Can you work these out from the model? Positions are in its coordinate system, mm. A direction names the side the tool comes from. Coordinates: 2 decimals unless noted, no trailing zeros. Order: outer loops, then holes, each group sorted by start corner. A loop starts at its lowest first (then second) coordinate and runs counter-clockwise, first axis right, second up. Notation, with made-up numbers: (-37.5, 54) -> (10.5, 54) arc R29 ccw to (10.5, 74) -> close; hole circle Ø11 at (63, 38.5). An arc over 180 degrees is marked (long way). Answer in a Markdown table with one row per item. Add a question column.
1. Imagine slicing it at C-C on x = -34. Write out the boundary of the cut face in (y, z), plus the area to 3 significant figures.
2. We'd pull the mould along Y, two halves only. Please class faces 1 (the face through (-22.185, -10.345, 0.21)), 2 (the face through (3.054, 2.707, 5.088)), 3 (the face through (-27, -18, 0)): pulls with the +Y half, pulls with the -Y half, needs draft (parallel to the pull), parting line crosses it, or undercut.
3. Imagine slicing it at B-B on y = 10. Write out the boundary of the cut face in (x, z), plus the area to 3 significant figures.
4. Will these pins go through, and if not, where does the flat tip stop? pin 1 (1.5 mm diameter, centred on x = -3, z = 3, fed in from +Y); pin 2 (5 mm diameter, centred on y = 14.71, z = -5, fed in from -X); pin 3 (3 mm diameter, centred on x = -12, y = -3.5, fed in from -Z); pin 4 (5 mm diameter, centred on y = -4.5, z = -2.5, fed in from -X).
5. If I drill on line 1 along X through (y, z) = (1, -10); line 2 along Z through (x, y) = (-25, -17.15); line 3 along Y through (x, z) = (-13.5, 12.5), over which ranges is the centre line in solid material (lowest first)? Write a range as [from, to].
6. Imagine slicing it at A-A on z = -10.25. Write out the boundary of the cut face in (x, y).
7. On a 3-axis mill with a long thin cutter (end or side, diameter ignored), from which of +Z, -Z, +X, -X, +Y, -Y can I reach the whole of each face in a straight line? I mean faces 4 (the face through (-9, -8, -15)), 5 (the face through (-4.53, -9.83, 6.77)), 6 (the face through (0, -18, 2)). Say none if no direction works.
from build123d import *

# Parameters (mm, degrees)
BOSS_EXTRUDE1_DEPTH             = 15
F_4_0MM_DOWEL_HOLE1_D           = 4
F_4_0MM_DOWEL_HOLE1_DEPTH       = 6
F_4_0MM_DOWEL_HOLE1_CSINK_D     = 4.05
F_4_0MM_DOWEL_HOLE1_CSINK_ANGLE = 90
F_4_0MM_DOWEL_HOLE1_TIP         = 1.201721238
F_4_0MM_DOWEL_HOLE3_D           = 4
F_4_0MM_DOWEL_HOLE3_DEPTH       = 6
F_4_0MM_DOWEL_HOLE3_CSINK_D     = 4.05
F_4_0MM_DOWEL_HOLE3_CSINK_ANGLE = 90
F_4_0MM_DOWEL_HOLE3_TIP         = 1.201721238


# Read off the part's stored shape, not the designer's step: Ø4.0mm Dowel Hole4
with BuildPart() as part:
    # Sketch1 → Boss-Extrude1 (new, symmetric)
    with BuildSketch(Plane.XY):
        Polygon((0, 19.016155383), (0, 0), (-45, -20.983844617), (7, -20.983844617), (7, 19.016155383), align=None)
    extrude(amount=BOSS_EXTRUDE1_DEPTH, both=True)

    # Ø4.0mm Dowel Hole1
    with Locations(Plane(origin=(0, -20.983844617, 0), x_dir=(-1, 0, 0), z_dir=(0, -1, 0))):
        with Locations((0, 0), (25, 0)):
            CounterSinkHole(F_4_0MM_DOWEL_HOLE1_D / 2, F_4_0MM_DOWEL_HOLE1_CSINK_D / 2, depth=F_4_0MM_DOWEL_HOLE1_DEPTH, counter_sink_angle=F_4_0MM_DOWEL_HOLE1_CSINK_ANGLE)
            with Locations((0, 0, -(F_4_0MM_DOWEL_HOLE1_DEPTH + F_4_0MM_DOWEL_HOLE1_TIP / 2))):  # 118° drill point
                Cone(0, F_4_0MM_DOWEL_HOLE1_D / 2, F_4_0MM_DOWEL_HOLE1_TIP, mode=Mode.SUBTRACT)

    # Ø4.0mm Dowel Hole3
    with Locations(Plane(origin=(0, 0, 0), x_dir=(0.9063077870366525, 0.422618261740694, 0), z_dir=(-0.422618261740694, 0.9063077870366525, 0))):
        with Locations((-23, 7), (-8, 7), (-8, -7), (-23, -7)):
            CounterSinkHole(F_4_0MM_DOWEL_HOLE3_D / 2, F_4_0MM_DOWEL_HOLE3_CSINK_D / 2, depth=F_4_0MM_DOWEL_HOLE3_DEPTH, counter_sink_angle=F_4_0MM_DOWEL_HOLE3_CSINK_ANGLE)
            with Locations((0, 0, -(F_4_0MM_DOWEL_HOLE3_DEPTH + F_4_0MM_DOWEL_HOLE3_TIP / 2))):  # 118° drill point
                Cone(0, F_4_0MM_DOWEL_HOLE3_D / 2, F_4_0MM_DOWEL_HOLE3_TIP, mode=Mode.SUBTRACT)

    # Ø4.0mm Dowel Hole4 outline → Ø4.0mm Dowel Hole4 (revolve, cut)
    with BuildSketch(Plane(origin=(0, 4.705485654, 5), x_dir=(0, 1, 0), z_dir=(0, 0, -1))):
        Polygon((0, 0), (2.025, 0), (2, 0.025), (2, 6), (0.335720518, 7), (0, 7), align=None)
    revolve(axis=Axis((0, 4.705485654, 5), (1, 0, 0)), mode=Mode.SUBTRACT)

    # 4.0mm Dowel Hole4 2 outline → 4.0mm Dowel Hole4 2 (revolve, cut)
    with BuildSketch(Plane(origin=(0, 14.705485654, -5), x_dir=(0, 1, 0), z_dir=(0, 0, -1))):
        Polygon((0, 0), (2.025, 0), (2, 0.025), (2, 6), (0.335720518, 7), (0, 7), align=None)
    revolve(axis=Axis((0, 14.705485654, -5), (1, 0, 0)), mode=Mode.SUBTRACT)

    # 4.0mm Dowel Hole4 3 outline → 4.0mm Dowel Hole4 3 (revolve, cut)
    with BuildSketch(Plane(origin=(0, 4.705485654, -5), x_dir=(0, 1, 0), z_dir=(0, 0, -1))):
        Polygon((0, 0), (2.025, 0), (2, 0.025), (2, 6), (0.335720518, 7), (0, 7), align=None)
    revolve(axis=Axis((0, 4.705485654, -5), (1, 0, 0)), mode=Mode.SUBTRACT)

    # 4.0mm Dowel Hole4 4 outline → 4.0mm Dowel Hole4 4 (revolve, cut)
    with BuildSketch(Plane(origin=(0, 14.705485654, 5), x_dir=(0, 1, 0), z_dir=(0, 0, -1))):
        Polygon((0, 0), (2.025, 0), (2, 0.025), (2, 6), (0.335720518, 7), (0, 7), align=None)
    revolve(axis=Axis((0, 14.705485654, 5), (1, 0, 0)), mode=Mode.SUBTRACT)


solid = part.part
Answers follow:
| question | item | result |
|---|---|---|
| 1 | outline | (-20.98, -15) -> (-15.85, -15) -> (-15.85, 15) -> (-20.98, 15) -> close |
| 1 | area | 154 mm² |
| 2 | face 1 | pulls with the +Y half |
| 2 | face 2 | undercut |
| 2 | face 3 | needs draft |
| 3 | outline | (0, -15) -> (7, -15) -> (7, 15) -> (0, 15) -> close |
| 3 | area | 210 mm² |
| 4 | pin 1 | stops at y = -1.05 |
| 4 | pin 2 | stops at x = 0 |
| 4 | pin 3 | passes through |
| 4 | pin 4 | stops at x = -15.01 |
| 5 | line 1 | x = [0, 7] |
| 5 | line 2 | z = [-15, -2], [2, 15] |
| 5 | line 3 | y = [-20.98, -6.3] |
| 6 | outline | (-45, -20.98) -> (7, -20.98) -> (7, 19.02) -> (0, 19.02) -> (0, 0) -> close |
| 7 | face 4 | -Z, +X, -X, +Y, -Y |
| 7 | face 5 | none |
| 7 | face 6 | -Y |
